Here's how the part is built. I have some questions about the finished solid (model axes, mm). A direction names the side the tool comes from. Give positions to 0.01 mm unless a question says otherwise; leave off trailing zeros. One line per item, written item: value. Start each with the question number.
```python
from build123d import *

# Parameters (mm, degrees)
SKETCH_1_W             = 23.5
SKETCH_1_H             = 12
EXTRUDE_1_DEPTH        = 650.5
HOLE_WIZARD_M6_1_D     = 5
HOLE_WIZARD_M6_1_DEPTH = 19
HOLE_WIZARD_M6_1_TIP   = 1.502151548
HOLE_WIZARD_M6_2_D     = 5
HOLE_WIZARD_M6_2_DEPTH = 19
HOLE_WIZARD_M6_2_TIP   = 1.502151548
HOLE_WIZARD_M4_1_D     = 3.3
HOLE_WIZARD_M4_1_DEPTH = 15.5
HOLE_WIZARD_M4_1_TIP   = 0.991420021
HOLE_WIZARD_9_0_9_1_D  = 9
HOLE_WIZARD_M4_2_D     = 3.3
HOLE_WIZARD_M4_2_DEPTH = 15.5
HOLE_WIZARD_M4_2_TIP   = 0.991420021


with BuildPart() as part:
    # 草图1 → 凸台-拉伸1 (new, symmetric)
    with BuildSketch(Plane(origin=(0, 0, 0), x_dir=(0, 0, -1), z_dir=(1, 0, 0))):
        Polygon((-15, 15), (-11.5, 15), (-11.5, 13.5), (-11, 13.5), (-11, 12), (-9.5, 12), (-9.5, 15), (-8, 15), (-8, 12.5), (-5, 12.5), (-5, 15), (5, 15), (5, 12.5), (8, 12.5), (8, 15), (9.5, 15), (9.5, 12), (11, 12), (11, 13.5), (11.5, 13.5), (11.5, 15), (15, 15), (15, 8), (12.5, 8), (12.5, 5), (15, 5), (15, -5), (12.5, -5), (12.5, -8), (15, -8), (15, -15), (11.5, -15), (11.5, -13.5), (11, -13.5), (11, -12), (9.5, -12), (9.5, -15), (8, -15), (8, -12.5), (5, -12.5), (5, -15), (-5, -15), (-5, -12.5), (-8, -12.5), (-8, -15), (-9.5, -15), (-9.5, -12), (-11, -12), (-11, -13.5), (-11.5, -13.5), (-11.5, -15), (-15, -15), align=None)
        with BuildLine():
            Line((12, -10.5), (12, -8.5))
            ThreePointArc((12, -8.5), (11.853553391, -8.146446609), (11.5, -8))
            Line((11.5, -8), (-11.5, -8))
            ThreePointArc((-11.5, -8), (-11.853553391, -8.146446609), (-12, -8.5))
            Line((-12, -8.5), (-12, -10.5))
            ThreePointArc((-12, -10.5), (-11.853553391, -10.853553391), (-11.5, -11))
            Line((-11.5, -11), (11.5, -11))
            ThreePointArc((11.5, -11), (11.853553391, -10.853553391), (12, -10.5))
        make_face(mode=Mode.SUBTRACT)
        with BuildLine():
            Line((-11.5, 11), (11.5, 11))
            ThreePointArc((11.5, 11), (11.853553391, 10.853553391), (12, 10.5))
            Line((12, 10.5), (12, 8.5))
            ThreePointArc((12, 8.5), (11.853553391, 8.146446609), (11.5, 8))
            Line((11.5, 8), (-11.5, 8))
            ThreePointArc((-11.5, 8), (-11.853553391, 8.146446609), (-12, 8.5))
            Line((-12, 8.5), (-12, 10.5))
            ThreePointArc((-12, 10.5), (-11.853553391, 10.853553391), (-11.5, 11))
        make_face(mode=Mode.SUBTRACT)
        Rectangle(SKETCH_1_W, SKETCH_1_H, mode=Mode.SUBTRACT)
    extrude(amount=EXTRUDE_1_DEPTH, both=True)

    # M6 螺纹孔1
    with Locations(Plane(origin=(0, -15, 0), x_dir=(-1, 0, 0), z_dir=(0, -1, 0))):
        with Locations((630.5, 0), (615.5, 0), (-615.5, 0), (-630.5, 0)):
            Hole(HOLE_WIZARD_M6_1_D / 2, depth=HOLE_WIZARD_M6_1_DEPTH)
            with Locations((0, 0, -(HOLE_WIZARD_M6_1_DEPTH + HOLE_WIZARD_M6_1_TIP / 2))):  # 118° drill point
                Cone(0, HOLE_WIZARD_M6_1_D / 2, HOLE_WIZARD_M6_1_TIP, mode=Mode.SUBTRACT)

    # M6 螺纹孔2
    with Locations(Plane(origin=(0, 0, -15), x_dir=(-1, 0, 0), z_dir=(0, 0, -1))):
        with Locations((-630.5, 0), (-615.5, 0), (630.5, 0), (615.5, 0)):
            Hole(HOLE_WIZARD_M6_2_D / 2, depth=HOLE_WIZARD_M6_2_DEPTH)
            with Locations((0, 0, -(HOLE_WIZARD_M6_2_DEPTH + HOLE_WIZARD_M6_2_TIP / 2))):  # 118° drill point
                Cone(0, HOLE_WIZARD_M6_2_D / 2, HOLE_WIZARD_M6_2_TIP, mode=Mode.SUBTRACT)

    # M4 螺纹孔1
    with Locations(Plane(origin=(0, -15, 0), x_dir=(-1, 0, 0), z_dir=(0, -1, 0))):
        with Locations((560, 0), (280, 0), (0, 0), (-280, 0), (-560, 0)):
            Hole(HOLE_WIZARD_M4_1_D / 2, depth=HOLE_WIZARD_M4_1_DEPTH)
            with Locations((0, 0, -(HOLE_WIZARD_M4_1_DEPTH + HOLE_WIZARD_M4_1_TIP / 2))):  # 118° drill point
                Cone(0, HOLE_WIZARD_M4_1_D / 2, HOLE_WIZARD_M4_1_TIP, mode=Mode.SUBTRACT)

    # Ø9.0 (9) 直径孔1 (through all)
    with Locations(Plane.XY.offset(15)):
        with Locations((525.5, 0), (-525.5, 0)):
            Hole(HOLE_WIZARD_9_0_9_1_D / 2)

    # M4 螺纹孔2
    with Locations(Plane(origin=(0, 0, -15), x_dir=(-1, 0, 0), z_dir=(0, 0, -1))):
        with Locations((-460, 0), (-230, 0), (0, 0), (230, 0), (460, 0), (-511.5, 0), (-539.5, 0), (539.5, 0), (511.5, 0)):
            Hole(HOLE_WIZARD_M4_2_D / 2, depth=HOLE_WIZARD_M4_2_DEPTH)
            with Locations((0, 0, -(HOLE_WIZARD_M4_2_DEPTH + HOLE_WIZARD_M4_2_TIP / 2))):  # 118° drill point
                Cone(0, HOLE_WIZARD_M4_2_D / 2, HOLE_WIZARD_M4_2_TIP, mode=Mode.SUBTRACT)


solid = part.part
```
(1) For faces 3 (the face through (9, 8, 0)), 4 (the face through (650.5, 7, 0)), which set-ups out of +Z, -Z, +X, -X, +Y, -Y let a thin tool reach every point of the face, with its end or its side?
(2) If we mould it in two halves opening along Y, with no side actions, what happens to faces 1 (the face through (9, 0, 15)), 2 (the face through (9, 11, 0))? For each: pulls with the +Y half, pulls with the -Y half, needs draft (parallel to the pull), parting line crosses it, or undercut.
(3) Will these pins go through, and if not, where does the flat tip stop? pin 1 (1.5 mm diameter, centred on x = -308, z = 6.5, fed in from -Y); pin 2 (10 mm diameter, centred on y = 2, z = 9.5, fed in from -X); pin 3 (2.5 mm diameter, centred on x = -539.5, y = 0, fed in from -Z); pin 4 (2.5 mm diameter, centred on x = -109.5, z = -6.5, fed in from +Y).
(4) Please list where these lines run through material, in increasing order: probe 1 along Y at (x, z) = (197, -4.75); probe 2 along Y at (x, z) = (-402, -6); probe 3 along Y at (x, z) = (-497, -13.25). Write a range as from..to.
(5) If we section it at A-A on x = -65.5: Give the number of separate pieces and of enclosed holes in the cut face, plus the area to 3 significant figures.
Found:
1. face 3: +X, -X
1. face 4: +Z, -Z, +X, +Y, -Y
2. face 1: needs draft
2. face 2: undercut
3. pin 1: y = -12.5
3. pin 2: x = -650.5
3. pin 3: z = 11.75
3. pin 4: y = 12.5
4. probe 1: -15..-11, -8..-6, 6..8, 11..15
4. probe 2: -12.5..-11, -8..-6, 6..8, 11..12.5
4. probe 3: -15..-8, -5..5, 8..15
5. separate pieces: 1
5. enclosed holes: 3
5. area: 408 mm^2
